```python
from build123d import *

# Parameters (mm, degrees)
F0_W                 = 30
F0_H                 = 20
F1_DEPTH             = 10
F4_D                 = 4.4
F4_DEPTH             = 14.4
F4_CBORE_D           = 8.25
F4_CBORE_DEPTH       = 4
F4_TIP               = 1.3218933619
F4_ON_F3_D           = 4.4
F4_ON_F3_DEPTH       = 14.4
F4_ON_F3_CBORE_D     = 8.25
F4_ON_F3_CBORE_DEPTH = 4
F4_ON_F3_TIP         = 1.3218933619
F6_D                 = 4
F6_DEPTH             = 10
F6_TIP               = 1.2017212381


with BuildPart() as f1:
    # F0 (on Top) → F1 (new body)
    with BuildSketch(Plane.XY):
        Polygon((-15, 50), (-35, 50), (-35, 0), (-10, 0), (-10, 20), (10, 20), (10, 0), (35, 0), (35, 50), (15, 50), align=None)
        with Locations((0, 60)):
            Rectangle(F0_W, F0_H)
    extrude(amount=F1_DEPTH)

    # F4
    with Locations(Plane.XZ):
        with Locations((-22.5, 5)):
            CounterBoreHole(F4_D / 2, F4_CBORE_D / 2, F4_CBORE_DEPTH, depth=F4_DEPTH)
            with Locations((0, 0, -(F4_DEPTH + F4_TIP / 2))):  # 118° drill point
                Cone(0, F4_D / 2, F4_TIP, mode=Mode.SUBTRACT)

    # F4 on F3
    with Locations(Plane.XZ):
        with Locations((22.5, 5)):
            CounterBoreHole(F4_ON_F3_D / 2, F4_ON_F3_CBORE_D / 2, F4_ON_F3_CBORE_DEPTH, depth=F4_ON_F3_DEPTH)
            with Locations((0, 0, -(F4_ON_F3_DEPTH + F4_ON_F3_TIP / 2))):  # 118° drill point
                Cone(0, F4_ON_F3_D / 2, F4_ON_F3_TIP, mode=Mode.SUBTRACT)

    # F6
    with Locations(Plane(origin=(0, 70, 0), x_dir=(-1, 0, 0), z_dir=(0, 1, 0))):
        with Locations((0, 5)):
            Hole(F6_D / 2, depth=F6_DEPTH)
            with Locations((0, 0, -(F6_DEPTH + F6_TIP / 2))):  # 118° drill point
                Cone(0, F6_D / 2, F6_TIP, mode=Mode.SUBTRACT)


solid = f1.part
```
The listing builds one solid part. Answer for the finished solid, in the listing's coordinates (mm). A direction names the side the tool comes from. Give positions to 0.01 mm unless a question says otherwise; leave off trailing zeros. Order: outer loops, then holes, each group sorted by start corner. A loop starts at its lowest first (then second) coordinate and runs counter-clockwise, first axis right, second up. Notation, with made-up numbers: (59.5, 82.25) -> (107.5, 82.25) arc R17 cw to (107.5, 112.25) -> close; hole circle Ø1 at (-29.5, 71). An arc over 180 degrees is marked (long way). Write each question's results on one line, items separated by ' | '.
Q1. Which of the six approach directions +Z, -Z, +X, -X, +Y, -Y give full straight-line access (tool end or side, diameter ignored) to faces 5 (the face through (-21, 4, 3)), 6 (the face through (25, 50, 5)), 7 (the face through (-25, 50, 5)), 8 (the face through (-10, 10, 5))?
Checked values:
face 5: -Y | face 6: +Z, -Z, +X, +Y | face 7: +Z, -Z, -X, +Y | face 8: +Z, -Z, -Y
Q2. The part is cut by section C-C, the plane x = 29. Give the vertices of the cut face in (y, z), and give its area (3 significant figures).
Checked values:
outline: (0, 0) -> (50, 0) -> (50, 10) -> (0, 10) -> close | area: 500 mm^2
Q3. Straight lines are drawn through the part: probe 1 along X at (y, z) = (66.5, 5); probe 2 along Z at (x, y) = (-22.5, 9.25); probe 3 along Z at (x, y) = (22.5, 1.45) (3 decimals). For each, find the intervals that lie inside material, in ascending order. Write a range as from..to.
Checked values:
probe 1: x = -15..-2, 2..15 | probe 2: z = 0..2.8, 7.2..10 | probe 3: z = 0..0.875, 9.125..10
Q4. Determine the mould class of faces 1 (the face through (-25.5, 0, 1.6)), 2 (the face through (22.197, 15.492, 4.768)), 3 (the face through (35, 25, 5)), 4 (the face through (-15, 60, 5)) for opening direction X: pulls with the +X half, pulls with the -X half, needs draft (parallel to the pull), parting line crosses it, or undercut.
Checked values:
face 1: needs draft | face 2: undercut | face 3: pulls with the +X half | face 4: pulls with the -X half
Q5. Each of these flat-tipped pins is pushed along its axis until it touches: P1, Ø1, axis at x = 8.5, z = 4.5, coming from the -Y side; P2, Ø1.5, axis at x = -21.5, z = 6.5, coming from the +Y side; P3, Ø5.5, axis at x = -22.5, z = 5, coming from the -Y side. Where does it stop, or does it pass through?
Checked values:
P1: stops at y = 20 | P2: stops at y = 50 | P3: stops at y = 4
Q6. The part is cut by section B-B, the plane y = 57. Give the vertices of the cut face in (x, z), and give its area (3 significant figures).
Checked values:
outline: (-15, 0) -> (15, 0) -> (15, 10) -> (-15, 10) -> close | area: 300 mm^2
Q7. The part is cut by section A-A, the plane y = 10.5. Give the vertices of the cut face in (x, z).
Checked values:
outline: (-35, 0) -> (-10, 0) -> (-10, 10) -> (-35, 10) -> close; (10, 0) -> (35, 0) -> (35, 10) -> (10, 10) -> close; hole circle Ø4.4 at (-22.5, 5); hole circle Ø4.4 at (22.5, 5)
